from build123d import *

# Parameters (mm, degrees)
SKETCH1_W               = 120
SKETCH1_H               = 65
BOSS_EXTRUDE1_DEPTH     = 30
CHAMFER1_SIZE           = 5
FILLET1_R               = 1.5
SHELL1_T                = -2.5
BOSS_EXTRUDE2_DEPTH     = 2
LPATTERN1_COUNT         = 2
LPATTERN1_PITCH         = 25
MIRROR1_COPY_1_DEPTH    = 2
BOSS_EXTRUDE3_DEPTH     = 2
BOSS_EXTRUDE4_DEPTH     = 2
CUT_EXTRUDE1_REACH      = 129.892
SKETCH7_R               = 6
SKETCH7_W               = 12
SKETCH7_H               = 8
CUT_EXTRUDE3_DEPTH      = 94.407708461
CUT_EXTRUDE3_DEPTH_BACK = 10
SKETCH9_R               = 3.25
CUT_EXTRUDE4_DEPTH      = 10
SKETCH6_R               = 3.2
SKETCH6_W               = 71.4
SKETCH6_H               = 24.65
CUT_EXTRUDE5_DEPTH      = 10


with BuildPart() as part:
    # Sketch1 → Boss-Extrude1 (new body)
    with BuildSketch(Plane(origin=(0, 0, 0), x_dir=(1, 0, 0), z_dir=(0, 1, 0))):
        Rectangle(SKETCH1_W, SKETCH1_H)
    extrude(amount=BOSS_EXTRUDE1_DEPTH)

    # Chamfer1
    chamfer1_edges = [part.edges().sort_by_distance(p)[0] for p in [
        (-60, 15, -32.5),
        (60, 15, -32.5),
        (60, 15, 32.5),
        (-60, 15, 32.5),
    ]]
    chamfer(chamfer1_edges, length=CHAMFER1_SIZE)

    # Fillet1
    fillet1_edges = [part.edges().sort_by_distance(p)[0] for p in [
        (0, 30, -32.5),
        (60, 30, 0),
        (-60, 30, 0),
        (0, 30, 32.5),
        (-57.5, 30, 30),
        (57.5, 30, 30),
        (-57.5, 30, -30),
        (57.5, 30, -30),
    ]]
    fillet(fillet1_edges, radius=FILLET1_R)

    # Shell1
    shell1_openings = [part.faces().sort_by_distance(p)[0] for p in [
        (0, 0, 0),
    ]]
    offset(amount=SHELL1_T, openings=shell1_openings, kind=Kind.INTERSECTION)

    # Sketch2 → Boss-Extrude2 (add, symmetric)
    with BuildSketch(Plane.XY.offset(20)):
        Polygon((47, 27.5), (47, 22), (40, 22), (40, 24), (37, 24), (37, 27.5), align=None)
    boss_extrude2 = extrude(amount=BOSS_EXTRUDE2_DEPTH, both=True)

    # LPattern1: Boss-Extrude2 ×2
    with Locations(*[(0, 0, -i * LPATTERN1_PITCH) for i in range(1, LPATTERN1_COUNT)]):
        add(boss_extrude2)

    # Mirror1: Boss-Extrude2 across plane
    add(boss_extrude2.mirror(Plane(origin=(0, 0, 0), x_dir=(0, 0, 1), z_dir=(1, 0, 0))))

    # Mirror1 copy 1 sketch → Mirror1 copy 1 (add, symmetric)
    with BuildSketch(Plane(origin=(0, 0, -5), x_dir=(-1, 0, 0), z_dir=(0, 0, 1))):
        Polygon((47, -27.5), (47, -22), (40, -22), (40, -24), (37, -24), (37, -27.5), align=None)
    extrude(amount=MIRROR1_COPY_1_DEPTH, both=True)

    # Sketch3 → Boss-Extrude3 (add, symmetric)
    with BuildSketch(Plane(origin=(32, 0, 0), x_dir=(0, 0, -1), z_dir=(1, 0, 0))):
        Polygon((17, 27.5), (17, 22), (10, 22), (10, 24), (7, 24), (7, 27.5), align=None)
        Polygon((-23, 27.5), (-30, 27.5), (-30, 22), (-26, 22), (-26, 24), (-23, 24), align=None)
    extrude(amount=BOSS_EXTRUDE3_DEPTH, both=True)

    # Sketch5 → Boss-Extrude4 (add, symmetric)
    with BuildSketch(Plane(origin=(-39.76, 0, 0), x_dir=(0, 0, -1), z_dir=(1, 0, 0))):
        Polygon((21.24, 27.5), (21.24, 20.25), (26.24, 20.25), (26.24, 17.75), (30, 17.75), (30, 27.5), align=None)
    extrude(amount=BOSS_EXTRUDE4_DEPTH, both=True)

    # Sketch7 → Cut-Extrude1 (cut, up to next)
    with BuildSketch(Plane.ZY.offset(60), mode=Mode.PRIVATE) as cut_extrude1_sk1:
        with Locations((19.3022, 14)):
            Circle(SKETCH7_R)
    cut_extrude1_tool1 = extrude(cut_extrude1_sk1.sketch, amount=-CUT_EXTRUDE1_REACH, mode=Mode.PRIVATE) & part.part
    # Sketch7 → Cut-Extrude1 (cut, up to next)
    with BuildSketch(Plane.ZY.offset(60), mode=Mode.PRIVATE) as cut_extrude1_sk2:
        with Locations((-12.5, 9)):
            Rectangle(SKETCH7_W, SKETCH7_H)
    cut_extrude1_tool2 = extrude(cut_extrude1_sk2.sketch, amount=-CUT_EXTRUDE1_REACH, mode=Mode.PRIVATE) & part.part
    add(cut_extrude1_tool1.solids().sort_by_distance((-60, 14, 19.3022))[0], mode=Mode.SUBTRACT)
    add(cut_extrude1_tool2.solids().sort_by_distance((-60, 9, -12.5))[0], mode=Mode.SUBTRACT)

    # Sketch8 → Cut-Extrude3 (cut, two sides: drawn at the far end of the back side and taken through both)
    with BuildSketch(Plane(origin=(0, 0, -32.5), x_dir=(-1, 0, 0), z_dir=(0, 0, -1)).offset(-CUT_EXTRUDE3_DEPTH_BACK)):
        with BuildLine():
            Line((-42, -234.178500307), (-42, 0))
            Line((-42, 0), (-42, 6))
            ThreePointArc((-42, 6), (-45, 9), (-48, 6))
            Line((-48, 6), (-48, 0))
            Line((-48, 0), (-48, -234.178500307))
            Line((-48, -234.178500307), (-48, -702.535500922))
            Line((-48, -702.535500922), (-42, -702.535500922))
            Line((-42, -702.535500922), (-42, -234.178500307))
        make_face()
    extrude(amount=CUT_EXTRUDE3_DEPTH + CUT_EXTRUDE3_DEPTH_BACK, mode=Mode.SUBTRACT)

    # Sketch9 → Cut-Extrude4 (cut)
    with BuildSketch(Plane.XY.offset(32.5)):
        with Locations((45, 15)):
            Circle(SKETCH9_R)
    extrude(amount=-CUT_EXTRUDE4_DEPTH, mode=Mode.SUBTRACT)

    # Sketch6 → Cut-Extrude5 (cut)
    with BuildSketch(Plane(origin=(0, 30, 0), x_dir=(1, 0, 0), z_dir=(0, 1, 0))):
        with Locations(Location((-29.52, 16.24, 0), (0, 0, 270))):
            Circle(SKETCH6_R)
        with Locations(Location((-19.36, 16.24, 0), (0, 0, 270))):
            Circle(SKETCH6_R)
        with Locations(Location((-4.12, 16.24, 0), (0, 0, 270))):
            Circle(SKETCH6_R)
        with Locations(Location((6.04, 16.24, 0), (0, 0, 270))):
            Circle(SKETCH6_R)
        with Locations((0, -8.475)):
            Rectangle(SKETCH6_W, SKETCH6_H)
    extrude(amount=-CUT_EXTRUDE5_DEPTH, mode=Mode.SUBTRACT)


solid = part.part
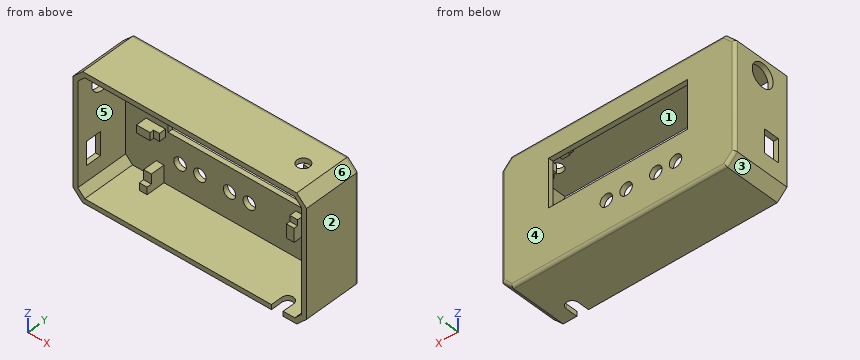
The model under review builds one solid part; all positions refer to its coordinate system, in mm. Face numbers are marked on the shaded views. A direction names the side the tool comes from. Round coordinates to 2 decimals unless told otherwise and drop trailing zeros. Loops run counter-clockwise (first coordinate to the right, second up) from the corner with the lowest first, then second, coordinate; pieces in that order, holes last. Notation, with made-up numbers: M -33,46 L -21,46 A15 cw -21,69 Z; hole C 57,65 d5. An arc over 180 degrees is marked long. Answer as CSV lines item,"result".
1. Insertion check: pin 1 Ø6 at (x, z) = (34.5, -7) entering from -Y; pin 2 Ø5 at (x, z) = (20, 1) entering from +Y; pin 3 Ø1.9 at (x, z) = (-40, -28) entering from -Y; pin 4 Ø3 at (x, z) = (-15.5, 19.5) entering from -Y. Each pin has a flat end and moves straight along its axis. Give the tip position at first contact, or say it passes through.
Outcome:
pin 1,"stops at y = 24"
pin 2,"passes through"
pin 3,"stops at y = 17.75"
pin 4,"stops at y = 27.5"
2. To check wall thickness, follow L1, parallel to X at y = 25.5, z = -12; L2, parallel to X at y = 28.6, z = -16.24; L3, parallel to X at y = 1.5, z = -15. State the ranges of each line that lie inside material, in increasing order. Write a range as [from, to].
Outcome:
L1,"x = [-60, -57.5], [30, 34], [57.5, 60]"
L2,"x = [-60, -32.72], [-26.32, -22.56], [-16.16, -7.32], [-0.92, 2.84], [9.24, 60]"
L3,"x = [-60, -57.5], [57.5, 60]"
3. We need section A-A (z = 5.5). Give the boundary of the cut face in (x, y).
Outcome:
outline,"M -60,0 L -57.5,0 L -57.5,27.5 L -35.7,27.5 L -35.7,30 L -58.5,30 A1.5 ccw -60,28.5 Z; M 35.7,27.5 L 57.5,27.5 L 57.5,0 L 60,0 L 60,28.5 A1.5 ccw 58.5,30 L 35.7,30 Z"
4. Draft analysis for pull direction X (two halves, no side actions). For the marked faces 3, 4, 5 and 6, state which applies: pulls with the +X half, pulls with the -X half, needs draft (parallel to the pull), parting line crosses it, or undercut.
Outcome:
face 3,"pulls with the -X half"
face 4,"needs draft"
face 5,"undercut"
face 6,"pulls with the +X half"
5. For the marked faces 1 and 2, list the 3-axis set-ups (+Z, -Z, +X, -X, +Y, -Y) from which the entire face can be reached by the end or side of a thin tool; tool diameter is ignored.
Outcome:
face 1,"-Y"
face 2,"+Z, -Z, +X, +Y, -Y"
6. We need section B-B (x = -19.36). Give the boundary of the cut face in (y, z).
Outcome:
outline,"M 0,-32.5 L 28.5,-32.5 A1.5 ccw 30,-31 L 30,-19.44 L 27.5,-19.44 L 27.5,-30 L 0,-30 Z; M 0,30 L 27.5,30 L 27.5,20.8 L 30,20.8 L 30,31 A1.5 ccw 28.5,32.5 L 0,32.5 Z; M 27.5,-13.04 L 30,-13.04 L 30,-3.85 L 27.5,-3.85 Z"
